Could you check a few things on this model? Use its own coordinates, in mm. A direction names the side the tool comes from. Coordinates: 2 decimals unless noted, no trailing zeros. Order: outer loops, then holes, each group sorted by start corner. A loop starts at its lowest first (then second) coordinate and runs counter-clockwise, first axis right, second up. Notation, with made-up numbers: (-25.5, 63.5) -> (-0.5, 63.5) arc R22 cw to (-0.5, 90.5) -> close; hole circle Ø9 at (-26, 34.5). An arc over 180 degrees is marked (long way). Put each result on its own line as item: value. Start each with the question number.
Q1. We'd pull the mould along Z, two halves only. Please class faces 3 (the face through (-0.59, -2.54, -4.46)), 4 (the face through (2.3, 0, 2.3)), 5 (the face through (7.765, -1.065, -0.17)): +Z half, -Z half, draft (parallel to the pull), parting line (faces both ways), or undercut.
Q2. If we section it at C-C (y = -2.4): Please give me the cut outline in (x, z), and give its area (3 significant figures).
Q3. For faces 1 (the face through (-4.3, -2.1, -2.1)), 2 (the face through (-9.514, -1.037, 2.996)), which set-ups out of +Z, -Z, +X, -X, +Y, -Y let a thin tool reach every point of the face, with its end or its side?
Q4. Will this pin go through, and if not, where does the flat tip stop? pin 1 (1.5 mm diameter, centred on x = 1.5, y = -2, fed in from -Z).
Q5. Please list where these lines run through material, in increasing order: line 1 along Y through (x, z) = (-4.75, -5); line 2 along Z through (x, y) = (2, -1.45); line 3 along X through (y, z) = (-2.6, 1.25).
Q6. If we section it at A-A (z = 0): Count the separate pieces of the cut face and the enclosed holes in it, and give its area (3 significant figures).
Autodesk Inventor part; units mm, degrees
ref_plane "YZ Plane" through (0, 0, 0) normal (1, 0, 0) x (0, 1, 0)
ref_plane "XZ Plane" through (0, 0, 0) normal (0, 1, 0) x (-1, 0, 0)
ref_plane "XY Plane" through (0, 0, 0) normal (0, 0, 1) x (1, 0, 0)
sketch "Sketch1" plane through (0, 0, 0) normal (0, 1, 0) x (-1, 0, 0)
  circle A0 centre (0, 0) radius 9.975
  dimension "d0" = 19.95
extrude "Extrusion1" add sketch "Sketch1" against normal blind 2.1
sketch "Sketch2" plane through (0, -2.1, 0) normal (0, -1, 0) x (1, 0, 0)
  circle A0 centre (0, 0) radius 4.5
  dimension "d3" = 9
extrude "Extrusion2" add sketch "Sketch2" along normal blind 1
sketch "Sketch3" plane through (0, 0, 0) normal (0, 1, 0) x (1, 0, 0)
  circle A0 centre (0, 0) radius 3
  dimension "d6" = 6
extrude "Extrusion3" cut sketch "Sketch3" against normal through all
chamfer "Chamfer1" distance 0.1 angle 45 3 edges at (9.975, 0, 0) (9.975, -2.1, 0) (-4.5, -3.1, 0)
sketch "Sketch4" plane through (0, 0, 0) normal (0, 1, 0) x (1, 0, 0)
  circle A0 centre (0, 0) radius 7
  point P0 (-7, 0)
  point P1 (7, 0)
  point P2 (0, -7)
  point P3 (0, 7)
  dimension "d12" = 14
hole "Hole1" at (7, 0, 0) at (0, 0, 7) at (0, 0, -7) at (-7, 0, 0) direction (0, -1, 0) diameter 1.567 end through all
properties part number "Bottom Horn" material "Aluminum 6061"
The answers:
1. face 3: parting line
1. face 4: draft
1. face 5: undercut
2. outline: circle Ø9 at (0, 0); hole circle Ø6 at (0, 0)
2. area: 35.3 mm^2
3. face 1: -Y
3. face 2: +Y, -Y
4. pin 1: z = -9.95
5. line 1: -2.1 to 0
5. line 2: -9.77 to -2.24, 2.24 to 9.77
5. line 3: -4.32 to -2.73, 2.73 to 4.32
6. separate pieces: 4
6. enclosed holes: 0
6. area: 25.7 mm^2
